Can you work these out from the model? Positions are in its coordinate system, mm. A direction names the side the tool comes from. Give positions to 0.01 mm unless a question says otherwise; leave off trailing zeros. Loops run counter-clockwise (first coordinate to the right, second up) from the corner with the lowest first, then second, coordinate; pieces in that order, holes last. Notation, with made-up numbers: (-25.75, 12.25) - (26.25, 12.25) arc R20 cw to (26.25, 26.25) - close; hole circle Ø4 at (38, 39.25). An arc over 180 degrees is marked (long way). Answer in a Markdown table with one row per item.
from build123d import *

# Parameters (mm, degrees)
ESQUISSE2_R             = 2.75
BOSS_EXTRU_1_DEPTH      = 20
ESQUISSE3_R             = 2.5
ENL_V_MAT_EXTRU_1_DEPTH = 20
ESQUISSE4_R             = 5
ESQUISSE4_R_2           = 2.75
ENL_V_MAT_EXTRU_2_DEPTH = 17


with BuildPart() as part:
    # Esquisse2 → Boss.-Extru.1 (new body)
    with BuildSketch(Plane(origin=(0, 0, 0), x_dir=(1, 0, 0), z_dir=(0, 1, 0))):
        with BuildLine():
            Line((-6.5, 0), (-27.5, 0))
            ThreePointArc((-27.5, 0), (-29.267766953, -0.732233047), (-30, -2.5))
            Line((-30, -2.5), (-30, -15))
            Line((-30, -15), (30, -15))
            Line((30, -15), (30, -2.5))
            ThreePointArc((30, -2.5), (29.267766953, -0.732233047), (27.5, 0))
            Line((27.5, 0), (6.5, 0))
            ThreePointArc((6.5, 0), (0, 6.5), (-6.5, 0))
        make_face()
        with Locations(Location((0, 0, 0), (0, 0, 270))):
            Circle(ESQUISSE2_R, mode=Mode.SUBTRACT)
    extrude(amount=BOSS_EXTRU_1_DEPTH)

    # Esquisse3 → Enlèv. mat.-Extru.1 (cut)
    with BuildSketch(Plane(origin=(0, 0, 0), x_dir=(-1, 0, 0), z_dir=(0, 0, -1))):
        with Locations((-20, 10)):
            Circle(ESQUISSE3_R)
        with Locations((20, 10)):
            Circle(ESQUISSE3_R)
    extrude(amount=-ENL_V_MAT_EXTRU_1_DEPTH, mode=Mode.SUBTRACT)

    # Esquisse4 → Enlèv. mat.-Extru.2 (cut)
    with BuildSketch(Plane.XZ):
        with Locations(Location((0, 0, 0), (0, 0, 270))):
            Circle(ESQUISSE4_R)
        with Locations(Location((0, 0, 0), (0, 0, 270))):
            Circle(ESQUISSE4_R_2, mode=Mode.SUBTRACT)
    extrude(amount=-ENL_V_MAT_EXTRU_2_DEPTH, mode=Mode.SUBTRACT)


solid = part.part
Q1. Imagine slicing it at A-A, the plane y = 10. Write out the boundary of the cut face in (x, z), and give its area (3 significant figures).
Checked values:
| item | result |
|---|---|
| outline | (-30, 2.5) arc R2.5 ccw to (-27.5, 0) - (-22.5, 0) - (-22.5, 15) - (-30, 15) - close; (-17.5, 0) - (-6.5, 0) arc R6.5 ccw to (6.5, 0) - (17.5, 0) - (17.5, 15) - (-17.5, 15) - close; (22.5, 0) - (27.5, 0) arc R2.5 ccw to (30, 2.5) - (30, 15) - (22.5, 15) - close; hole circle Ø10 at (0, 0) |
| area | 735 mm² |
Q2. On a 3-axis mill with a long thin cutter (end or side, diameter ignored), from which of +Z, -Z, +X, -X, +Y, -Y can I reach the whole of each face in a straight line? I mean faces 1 (the face through (-17, 10, 0)), 2 (the face through (0.1, 9.9, -6.5)), 3 (the face through (-4.88, 8.38, 1.08)). Say none if no direction works.
Checked values:
| item | result |
|---|---|
| face 1 | -Z, -X, +Y, -Y |
| face 2 | -Z, +Y, -Y |
| face 3 | -Y |
Q3. If I drill on line 1 (Z direction, x = 0, y = 19.3); line 2 (Y direction, x = 20, z = 7.25); line 3 (Z direction, x = -8.5, y = 8.5), over which ranges is the centre line in solid material (lowest first)? Write a range as [from, to].
Checked values:
| item | result |
|---|---|
| line 1 | z = [-6.5, -2.75], [2.75, 15] |
| line 2 | y = [0, 7.5], [12.5, 20] |
| line 3 | z = [0, 15] |
Q4. Imagine slicing it at C-C, the plane y = 2.25. Write out the boundary of the cut face in (x, z).
Checked values:
| item | result |
|---|---|
| outline | (-30, 2.5) arc R2.5 ccw to (-27.5, 0) - (-6.5, 0) arc R6.5 ccw to (6.5, 0) - (27.5, 0) arc R2.5 ccw to (30, 2.5) - (30, 15) - (-30, 15) - close; hole circle Ø10 at (0, 0) |
Q5. Imagine slicing it at B-B, the plane x = -20. Write out the boundary of the cut face in (y, z).
Checked values:
| item | result |
|---|---|
| outline | (0, 0) - (7.5, 0) - (7.5, 15) - (0, 15) - close; (12.5, 0) - (20, 0) - (20, 15) - (12.5, 15) - close |
Q6. Imagine slicing it at D-D, the plane z = 8.5. Write out the boundary of the cut face in (x, y), and give its area (3 significant figures).
Checked values:
| item | result |
|---|---|
| outline | (-30, 0) - (30, 0) - (30, 20) - (-30, 20) - close; hole circle Ø5 at (-20, 10); hole circle Ø5 at (20, 10) |
| area | 1,160 mm² |
Q7. If we mould it in two halves opening along X, with no side actions, what happens to faces 4 (the face through (-30, 10, 9)), 5 (the face through (17, 10, 0)), 6 (the face through (-2.2, 17, -2.2))? For each: released by +X, released by -X, zero draft, split by the parting line, or undercut.
Checked values:
| item | result |
|---|---|
| face 4 | released by -X |
| face 5 | zero draft |
| face 6 | undercut |
Q8. For pin 1 (3.5 mm diameter, centred on x = 0, z = 0, fed in from -Y), with a flat end and sliding along its axis, tell me the tip position at first contact or that it passes through.
Checked values:
| item | result |
|---|---|
| pin 1 | passes through |
